Answer from the drawing. Dimensions are ordinates in mm from the lowest x, y and z of the part. A direction names the side the tool comes from. Round coordinates to 2 decimals unless told otherwise and drop trailing zeros. Write each loop counter-clockwise with the first axis right and the second up, starting at its lowest first coordinate (ties: lowest second). Pieces come first, ordered by that corner, then holes. Notation, with made-up numbers: (-34, 86.25) - (-29, 86.25) arc R24 ccw to (-29, 125.25) - close; hole circle Ø5 at (56, -15.75). An arc over 180 degrees is marked (long way). Answer in a Markdown table with one row per item.
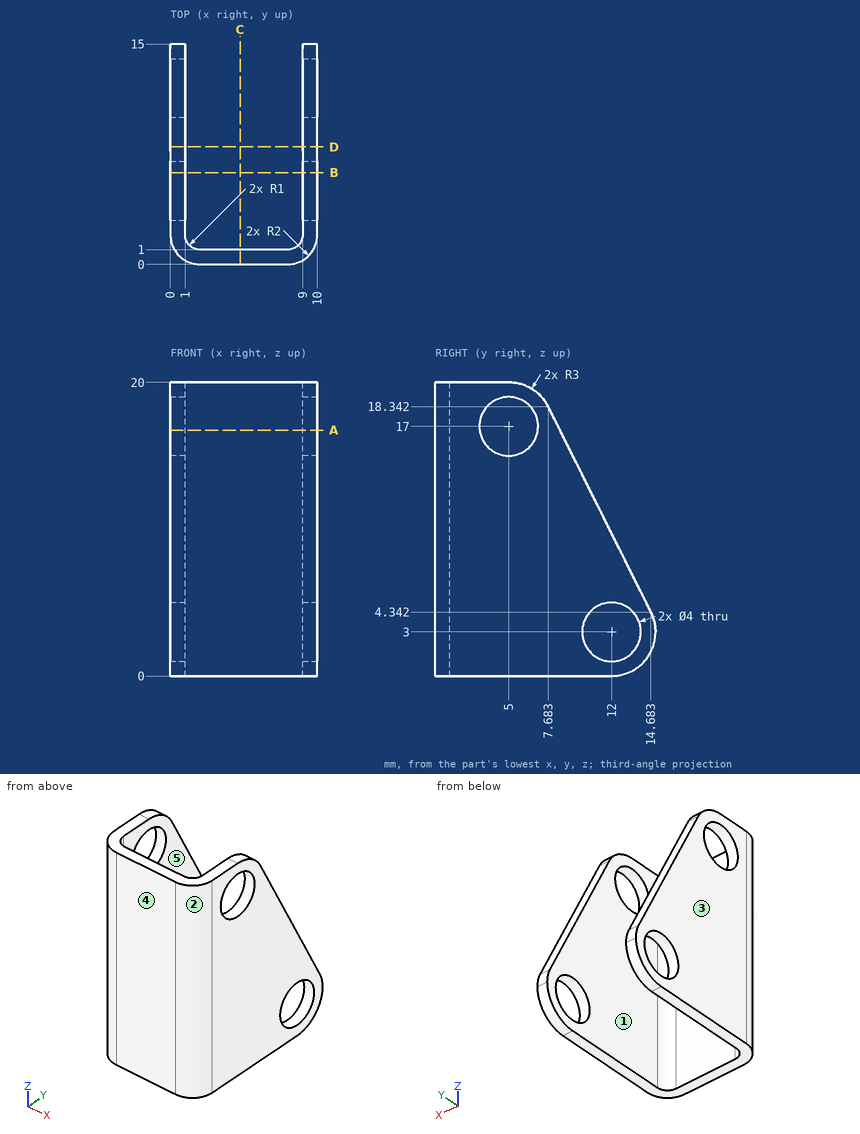
(1) Section C-C (x = 4.75) is taken. Give the vertices of the cut face in (y, z), and give its area (3 significant figures).
Checked values:
| item | result |
|---|---|
| outline | (0, 0) - (1, 0) - (1, 20) - (0, 20) - close |
| area | 20.0 mm2 |
(2) Find the intervals of material crossed by line 1 (X direction, y = 4.75, z = 11.75); line 2 (Y direction, x = 4.5, z = 3.5); line 3 (Y direction, x = 0.7, z = 17) (1 decimal), in increasing order.
Checked values:
| item | result |
|---|---|
| line 1 | x = 0 to 1, 9 to 10 |
| line 2 | y = 0 to 1 |
| line 3 | y = 0.5 to 3, 7 to 8.4 |
(3) For a pull along X with two mould halves and no side action, classify the marked faces 3, 4 and 5 as pulls with the +X half, pulls with the -X half, needs draft (parallel to the pull), parting line crosses it, or undercut.
Checked values:
| item | result |
|---|---|
| face 3 | pulls with the -X half |
| face 4 | needs draft |
| face 5 | undercut |
(4) Section D-D (y = 8) is taken. Give the vertices of the cut face in (x, z).
Checked values:
| item | result |
|---|---|
| outline | (0, 0) - (1, 0) - (1, 17.71) - (0, 17.71) - close; (9, 0) - (10, 0) - (10, 17.71) - (9, 17.71) - close |
(5) Flat-ended cylindrical pins translate along their axes: pin 1 (3.5 mm diameter, centred on y = 5, z = 17, fed in from -X); pin 2 (1 mm diameter, centred on x = 5.5, z = 11.5, fed in from +Y); pin 3 (3 mm diameter, centred on x = 2, y = 8, fed in from +Z) (1 decimal); pin 4 (2 mm diameter, centred on x = 1.5, z = 8.5, fed in from +Y). Find the tip coordinate at first contact, or state that the pin passes through.
Checked values:
| item | result |
|---|---|
| pin 1 | passes through |
| pin 2 | stops at y = 1 |
| pin 3 | stops at z = 19.3 |
| pin 4 | stops at y = 13.04 |
(6) For the marked faces 1 and 2, determine the directions among +Z, -Z, +X, -X, +Y, -Y from which every point of the face is accessible in a straight line to the end or side of a thin tool.
Checked values:
| item | result |
|---|---|
| face 1 | +Z, -Z, +Y |
| face 2 | +Z, -Z, +X, -Y |
(7) Section A-A (z = 16.75) is taken. Give the vertices of the cut face in (x, y) (1 decimal).
Checked values:
| item | result |
|---|---|
| outline | (0, 2) arc R2 ccw to (2, 0) - (8, 0) arc R2 ccw to (10, 2) - (10, 3) - (9, 3) - (9, 2) arc R1 cw to (8, 1) - (2, 1) arc R1 cw to (1, 2) - (1, 3) - (0, 3) - close; (0, 7) - (1, 7) - (1, 8.5) - (0, 8.5) - close; (9, 7) - (10, 7) - (10, 8.5) - (9, 8.5) - close |
(8) Section B-B (y = 6.25) is taken. Give the vertices of the cut face in (x, z).
Checked values:
| item | result |
|---|---|
| outline | (0, 0) - (1, 0) - (1, 15.44) - (0, 15.44) - close; (0, 18.56) - (1, 18.56) - (1, 19.73) - (0, 19.73) - close; (9, 0) - (10, 0) - (10, 15.44) - (9, 15.44) - close; (9, 18.56) - (10, 18.56) - (10, 19.73) - (9, 19.73) - close |
